Verification items for the finished model (mm, model axes). Give positions to 0.01 mm unless a question says otherwise; leave off trailing zeros. Order: outer loops, then holes, each group sorted by start corner. A loop starts at its lowest first (then second) coordinate and runs counter-clockwise, first axis right, second up. Notation, with made-up numbers: (41, 48.25) -> (51, 48.25) arc R13 cw to (51, 69.25) -> close; hole circle Ø10 at (65, -27.5). An arc over 180 degrees is marked (long way). One line per question, with ' | ' between items. Start each with the question number.
Q1. Material ranges on probe 1 along Y at (x, z) = (-17, 1.2); probe 2 along Y at (x, z) = (-90, 1); probe 3 along Y at (x, z) = (24, 1.4), recorded low to high. Write a range as [from, to].
Q2. Section check C-C on z = 0.3. Give the number of separate pieces and of enclosed holes in the cut face, plus the area to 3 significant figures.
Q3. Section check B-B on x = 24.5. Record the cut outline in (y, z), plus the area to 3 significant figures.
Q4. Section check A-A on x = -66. Record the cut outline in (y, z), plus the area to 3 significant figures.
Q5. Go/stop test with a flat-tipped pin: pin 1 (4 mm diameter, centred on x = -99, y = -34, fed in from +Z). Record where the tip stops, or that it passes through.
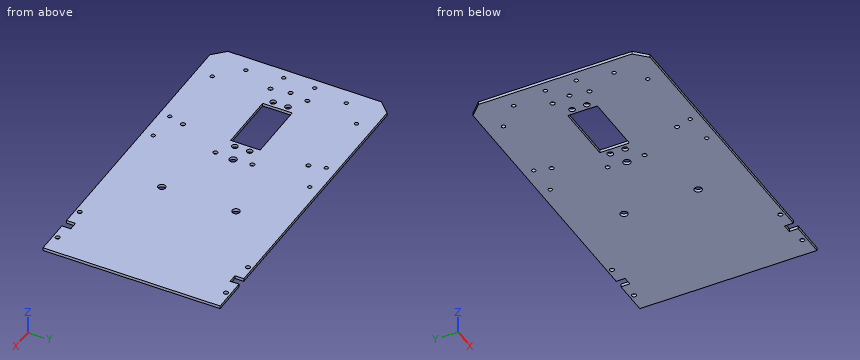
from build123d import *

# Parameters (mm, degrees)
SKETCH_5_W           = 220
SKETCH_5_H           = 120
EXTRUDE_2_DEPTH      = 2
SKETCH_6_R           = 2.5
CUT_EXTRUDE_3_DEPTH  = 126.315601583
SKETCH_7_R           = 1.5
SKETCH_7_W           = 6
SKETCH_7_H           = 6
CUT_EXTRUDE_4_DEPTH  = 126.315601583
SKETCH_9_R           = 2
SKETCH_9_W           = 40.7
SKETCH_9_H           = 20
CUT_EXTRUDE_6_DEPTH  = 126.315601583
SKETCH_13_R          = 1.3
CUT_EXTRUDE_10_DEPTH = 126.315601583
CHAMFER_1_SIZE       = 8
SKETCH_15_R          = 1.3
CUT_EXTRUDE_12_DEPTH = 126.315601583
SKETCH_16_R          = 1.3
CUT_EXTRUDE_13_DEPTH = 126.315601583
SKETCH_17_R          = 1.5
CUT_EXTRUDE_14_DEPTH = 126.315601583
SKETCH_19_R          = 1.5
CUT_EXTRUDE_15_DEPTH = 126.315601583


with BuildPart() as part:
    # 草图5 → 凸台-拉伸2 (new body)
    with BuildSketch(Plane.XY):
        Rectangle(SKETCH_5_W, SKETCH_5_H)
    extrude(amount=EXTRUDE_2_DEPTH)

    # 草图6 → 切除-拉伸3 (cut, through all)
    with BuildSketch(Plane.XY.offset(2)):
        with Locations((-19, 0)):
            Circle(SKETCH_6_R)
        with Locations((24.5, 25.11473671)):
            Circle(SKETCH_6_R)
        with Locations((24.5, -25.11473671)):
            Circle(SKETCH_6_R)
    extrude(amount=-CUT_EXTRUDE_3_DEPTH, mode=Mode.SUBTRACT)

    # 草图7 → 切除-拉伸4 (cut, through all)
    with BuildSketch(Plane.XY.offset(2)):
        with Locations((69, 57)):
            Circle(SKETCH_7_R)
        with Locations(Location((97, 57, 0), (0, 0, 180))):
            Circle(SKETCH_7_R)
        with Locations((97, -57)):
            Circle(SKETCH_7_R)
        with Locations(Location((69, -57, 0), (0, 0, 180))):
            Circle(SKETCH_7_R)
        with Locations((83, 57)):
            Rectangle(SKETCH_7_W, SKETCH_7_H)
        with Locations((83, -57)):
            Rectangle(SKETCH_7_W, SKETCH_7_H)
    extrude(amount=-CUT_EXTRUDE_4_DEPTH, mode=Mode.SUBTRACT)

    # 草图9 → 切除-拉伸6 (cut, through all)
    with BuildSketch(Plane.XY.offset(2)):
        with Locations((-79.315, 5)):
            Circle(SKETCH_9_R)
        with Locations(Location((-79.315, -5, 0), (0, 0, 180))):
            Circle(SKETCH_9_R)
        with Locations((-30.685, -5)):
            Circle(SKETCH_9_R)
        with Locations(Location((-30.685, 5, 0), (0, 0, 180))):
            Circle(SKETCH_9_R)
        with Locations((-55, 0)):
            Rectangle(SKETCH_9_W, SKETCH_9_H)
    extrude(amount=-CUT_EXTRUDE_6_DEPTH, mode=Mode.SUBTRACT)

    # 草图13 → 切除-拉伸10 (cut, through all)
    with BuildSketch(Plane.XY.offset(2)):
        with Locations((-103, 10.5)):
            Circle(SKETCH_13_R)
        with Locations(Location((-103, -10.5, 0), (0, 0, 180))):
            Circle(SKETCH_13_R)
    extrude(amount=-CUT_EXTRUDE_10_DEPTH, mode=Mode.SUBTRACT)

    # 倒角1
    chamfer_1_edges = [part.edges().sort_by_distance(p)[0] for p in [
        (-110, -60, 1),
        (-110, 60, 1),
    ]]
    chamfer(chamfer_1_edges, length=CHAMFER_1_SIZE)

    # 草图15 → 切除-拉伸12 (cut, through all)
    with BuildSketch(Plane.XY.offset(2)):
        with Locations((-38, 53)):
            Circle(SKETCH_15_R)
        with Locations(Location((-38, -53, 0), (0, 0, 180))):
            Circle(SKETCH_15_R)
        with Locations((-17, 53)):
            Circle(SKETCH_15_R)
        with Locations(Location((-17, -53, 0), (0, 0, 180))):
            Circle(SKETCH_15_R)
    extrude(amount=-CUT_EXTRUDE_12_DEPTH, mode=Mode.SUBTRACT)

    # 草图16 → 切除-拉伸13 (cut, through all)
    with BuildSketch(Plane.XY.offset(2)):
        with Locations((-99, 34)):
            Circle(SKETCH_16_R)
        with Locations((-84.150757595, 48.849242405)):
            Circle(SKETCH_16_R)
        with Locations(Location((-99, -34, 0), (0, 0, 180))):
            Circle(SKETCH_16_R)
        with Locations(Location((-84.150757595, -48.849242405, 0), (0, 0, 180))):
            Circle(SKETCH_16_R)
    extrude(amount=-CUT_EXTRUDE_13_DEPTH, mode=Mode.SUBTRACT)

    # 草图17 → 切除-拉伸14 (cut, through all)
    with BuildSketch(Plane.XY.offset(2)):
        with Locations((-20, 12.5)):
            Circle(SKETCH_17_R)
        with Locations(Location((-20, -12.5, 0), (0, 0, 180))):
            Circle(SKETCH_17_R)
        with Locations((-90, 12.5)):
            Circle(SKETCH_17_R)
        with Locations(Location((-90, -12.5, 0), (0, 0, 180))):
            Circle(SKETCH_17_R)
    extrude(amount=-CUT_EXTRUDE_14_DEPTH, mode=Mode.SUBTRACT)

    # 草图19 → 切除-拉伸15 (cut, through all)
    with BuildSketch(Plane.XY.offset(2)):
        with Locations((-92, 0)):
            Circle(SKETCH_19_R)
        with Locations((-35, 42.5)):
            Circle(SKETCH_19_R)
        with Locations(Location((-35, -42.5, 0), (0, 0, 180))):
            Circle(SKETCH_19_R)
    extrude(amount=-CUT_EXTRUDE_15_DEPTH, mode=Mode.SUBTRACT)


solid = part.part
Filled in:
1) probe 1: [-60, -54.3], [-51.7, -1.5], [1.5, 51.7], [54.3, 60] | probe 2: [-60, -14], [-11, 11], [14, 60] | probe 3: [-60, -27.56], [-22.67, 22.67], [27.56, 60]
2) separate pieces: 1 | enclosed holes: 29 | area: 25,200 mm²
3) outline: (-60, 0) -> (-27.61, 0) -> (-27.61, 2) -> (-60, 2) -> close; (-22.61, 0) -> (22.61, 0) -> (22.61, 2) -> (-22.61, 2) -> close; (27.61, 0) -> (60, 0) -> (60, 2) -> (27.61, 2) -> close | area: 220 mm²
4) outline: (-60, 0) -> (-10, 0) -> (-10, 2) -> (-60, 2) -> close; (10, 0) -> (60, 0) -> (60, 2) -> (10, 2) -> close | area: 200 mm²
5) pin 1: z = 2
